Design review of the part built by this model. Coordinates are the model's own, in mm. A direction names the side the tool comes from. Coordinates: 2 decimals unless noted, no trailing zeros. Loops run counter-clockwise (first coordinate to the right, second up) from the corner with the lowest first, then second, coordinate; pieces in that order, holes last. Notation, with made-up numbers: (73.25, 1) - (130.25, 1) arc R24 ccw to (130.25, 19) - close; hole circle Ø10 at (17.5, -26). An arc over 180 degrees is marked (long way). Use one line per item in the form item = value. Start each with the question number.
(1) Clearance check with flat-ended pins moving along their axes: pin 1 Ø1 at (x, z) = (-14, 0) entering from +Y; pin 2 Ø6 at (y, z) = (15, 9.5) entering from +X; pin 3 Ø4 at (y, z) = (3.5, 3.5) entering from -X. State where each tip first meets the part, or that it passes through.
(2) For L1, parallel to X at y = 19.15, z = 0; L2, parallel to Z at x = 0, y = 7.25; L3, parallel to Y at x = -0.5, z = 11, list the stretches that pass through material, from the lowest coordinate up.
(3) Tool access review of faces 5 (the face through (-17.847, 19.246, 2.343)), 6 (the face through (-0.35, 14.18, -0.11)): name each direction out of +Z, -Z, +X, -X, +Y, -Y from which nothing blocks a thin tool from reaching the whole face with its end or side.
(4) Add section B-B (y = 15.25). State the section outline as (x, z) points.
(5) The part is to be moulded in two halves that separate along X. For faces 1 (the face through (-4.3, 19, 8.3)), 2 (the face through (2.003, 6.871, -0.631)), 3 (the face through (19.524, 10.133, 4.336)), 4 (the face through (0, 20, 0)), say which applies: pulls with the +X half, pulls with the -X half, needs draft (parallel to the pull), parting line crosses it, or undercut.
(6) Add section A-A (y = 3.5). State the section outline as (x, z) points, plus the area to 3 significant figures.
```python
from build123d import *

# Parameters (mm, degrees)
CHAMFER1_SIZE                   = 0.5
M5X0_8_TAPPED_HOLE1_D           = 4.2
M5X0_8_TAPPED_HOLE1_DEPTH       = 13.1381927
M5X0_8_TAPPED_HOLE1_CSINK_D     = 5.05
M5X0_8_TAPPED_HOLE1_CSINK_ANGLE = 90
M5X0_8_TAPPED_HOLE1_TIP         = 1.2618073


with BuildPart() as part:
    # Sketch1 → Revolve1 (revolve)
    with BuildSketch(Plane(origin=(0, 0, 0), x_dir=(0, 0, -1), z_dir=(1, 0, 0))):
        Polygon((0, 0), (20, 0), (20, 20), (18, 20), (18, 19), (9, 19), (9, 20), (0, 20), align=None)
    revolve(axis=Axis((0, 0, 0), (0, 1, 0)))

    # Chamfer1
    chamfer1_edges = [part.edges().sort_by_distance(p)[0] for p in [
        (0, 20, 9),
        (0, 20, 18),
        (0, 20, 20),
        (0, 0, 20),
    ]]
    chamfer(chamfer1_edges, length=CHAMFER1_SIZE)

    # M5x0.8 Tapped Hole1
    with Locations(Plane(origin=(0, 0, 0), x_dir=(-1, 0, 0), z_dir=(0, -1, 0))):
        with Locations((0, 0)):
            CounterSinkHole(M5X0_8_TAPPED_HOLE1_D / 2, M5X0_8_TAPPED_HOLE1_CSINK_D / 2, depth=M5X0_8_TAPPED_HOLE1_DEPTH, counter_sink_angle=M5X0_8_TAPPED_HOLE1_CSINK_ANGLE)
            with Locations((0, 0, -(M5X0_8_TAPPED_HOLE1_DEPTH + M5X0_8_TAPPED_HOLE1_TIP / 2))):  # 118° drill point
                Cone(0, M5X0_8_TAPPED_HOLE1_D / 2, M5X0_8_TAPPED_HOLE1_TIP, mode=Mode.SUBTRACT)


solid = part.part
```
Computed values:
q1.pin_1 = 19
q1.pin_2 = 18.91
q1.pin_3 = -19.94
q2.L1 = -20 to -18, -9 to 9, 18 to 20
q2.L2 = -20 to -2.1, 2.1 to 20
q2.L3 = 0 to 19
q3.face_5 = +Y
q3.face_6 = -Y
q4.outline = circle Ø40 at (0, 0)
q5.face_1 = undercut
q5.face_2 = undercut
q5.face_3 = parting line crosses it
q5.face_4 = needs draft
q6.outline = circle Ø40 at (0, 0); hole circle Ø4.2 at (0, 0)
q6.area = 1,240 mm^2
